For this review, take the finished solid that the model builds, in its own axes (mm). Face numbers are marked on the shaded views. A direction names the side the tool comes from. Give positions to 0.01 mm unless a question says otherwise; leave off trailing zeros. Order: outer loops, then holes, each group sorted by start corner. A loop starts at its lowest first (then second) coordinate and runs counter-clockwise, first axis right, second up.
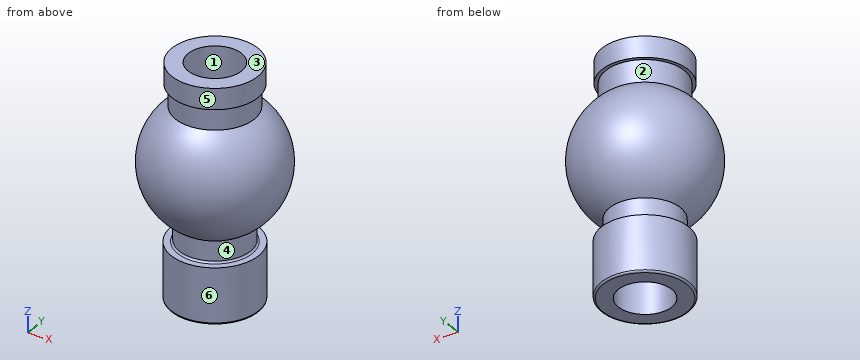
from build123d import *

# Parameters (mm, degrees)
SKETCH1_R           = 2.45
SKETCH1_R_2         = 1.5
BOSS_EXTRUDE1_DEPTH = 3.12
SKETCH2_R           = 1.99
SKETCH2_R_2         = 1.5
BOSS_EXTRUDE2_DEPTH = 1.2
FILLET1_R           = 0.1
CUT_EXTRUDE1_START  = -8.2
SKETCH5_R           = 1.5
CUT_EXTRUDE1_DEPTH  = 8.2
SKETCH6_R           = 2.21
SKETCH6_R_2         = 1.5
BOSS_EXTRUDE3_DEPTH = 1.24
SKETCH7_R           = 2.41
SKETCH7_R_2         = 1.5
BOSS_EXTRUDE4_DEPTH = 1.17


with BuildPart() as part:
    # Sketch1 → Boss-Extrude1 (new body)
    with BuildSketch(Plane.XY):
        with Locations(Location((0, 0, 0), (0, 0, 180))):
            Circle(SKETCH1_R)
        with Locations(Location((0, 0, 0), (0, 0, 180))):
            Circle(SKETCH1_R_2, mode=Mode.SUBTRACT)
    extrude(amount=BOSS_EXTRUDE1_DEPTH)

    # Sketch2 → Boss-Extrude2 (add)
    with BuildSketch(Plane.XY.offset(3.12)):
        Circle(SKETCH2_R)
        with Locations(Location((0, 0, 0), (0, 0, 180))):
            Circle(SKETCH2_R_2, mode=Mode.SUBTRACT)
    extrude(amount=BOSS_EXTRUDE2_DEPTH)

    # Fillet1
    fillet1_edges = [part.edges().sort_by_distance(p)[0] for p in [
        (-1.99, 0, 3.12),
        (2.45, 0, 0),
    ]]
    fillet(fillet1_edges, radius=FILLET1_R)

    # Sketch3 → Revolve1 (revolve)
    with BuildSketch(Plane(origin=(0, 0, 0), x_dir=(0, 0, -1), z_dir=(1, 0, 0))):
        with BuildLine():
            Line((-4.32, 0), (-4.32, 1.99))
            ThreePointArc((-4.32, 1.99), (-7.365617926, 3.747647485), (-10.528014715, 2.21))
            Line((-10.528014715, 2.21), (-10.528014715, 0))
            Line((-10.528014715, 0), (-4.32, 0))
        make_face()
    revolve(axis=Axis((0, 0, 4.32), (0, 0, 1)))

    # Sketch5 → Cut-Extrude1 (cut)
    with BuildSketch(Plane.XY.offset(10.528014715).offset(CUT_EXTRUDE1_START)):
        with Locations(Location((0, 0, 0), (0, 0, 180))):
            Circle(SKETCH5_R)
    extrude(amount=CUT_EXTRUDE1_DEPTH, mode=Mode.SUBTRACT)

    # Sketch6 → Boss-Extrude3 (add)
    with BuildSketch(Plane.XY.offset(10.528014715)):
        with Locations(Location((0, 0, 0), (0, 0, 90))):
            Circle(SKETCH6_R)
        with Locations(Location((0, 0, 0), (0, 0, 180))):
            Circle(SKETCH6_R_2, mode=Mode.SUBTRACT)
    extrude(amount=BOSS_EXTRUDE3_DEPTH)

    # Sketch7 → Boss-Extrude4 (add)
    with BuildSketch(Plane.XY.offset(11.768014715)):
        with Locations(Location((0, 0, 0), (0, 0, 180))):
            Circle(SKETCH7_R)
        with Locations(Location((0, 0, 0), (0, 0, 180))):
            Circle(SKETCH7_R_2, mode=Mode.SUBTRACT)
    extrude(amount=BOSS_EXTRUDE4_DEPTH)


solid = part.part
1) We need section A-A on y = 0. Give the boundary of the cut face in (x, z), then the cut area to 3 significant figures.
Answer sheet:
outline: (-2.45, 0.1) arc R0.1 ccw to (-2.35, 0) - (-1.5, 0) - (-1.5, 12.94) - (-2.41, 12.94) - (-2.41, 11.77) - (-2.21, 11.77) - (-2.21, 10.53) arc R3.75 ccw to (-1.99, 4.32) - (-1.99, 3.22) arc R0.1 cw to (-2.09, 3.12) - (-2.45, 3.12) - close; (1.5, 0) - (2.35, 0) arc R0.1 ccw to (2.45, 0.1) - (2.45, 3.12) - (2.09, 3.12) arc R0.1 cw to (1.99, 3.22) - (1.99, 4.32) arc R3.75 ccw to (2.21, 10.53) - (2.21, 11.77) - (2.41, 11.77) - (2.41, 12.94) - (1.5, 12.94) - close
area: 32.8 mm2
2) We need section D-D on z = 1.25. Give the boundary of the cut face in (x, y), then the cut area to 3 significant figures.
Answer sheet:
outline: circle Ø4.9 at (0, 0); hole circle Ø3 at (0, 0)
area: 11.8 mm2
3) To check wall thickness, follow line 1 (Z direction, x = -2, y = -0.75); line 2 (Y direction, x = -0.75, z = 1.75); line 3 (Y direction, x = 0, z = 5). State the ranges of each line that lie inside material, in increasing order.
Answer sheet:
line 1: z = 0 to 3.12, 4.42 to 12.94
line 2: y = -2.33 to -1.3, 1.3 to 2.33
line 3: y = -2.8 to -1.5, 1.5 to 2.8
4) Tool access review of the marked faces 4, 5 and 6: name each direction out of +Z, -Z, +X, -X, +Y, -Y from which nothing blocks a thin tool from reaching the whole face with its end or side.
Answer sheet:
face 4: none
face 5: +Z
face 6: -Z
5) We need section C-C on z = 12.25. Give the boundary of the cut face in (x, y).
Answer sheet:
outline: circle Ø4.82 at (0, 0); hole circle Ø3 at (0, 0)
6) Clearance check with flat-ended pins moving along their axes: pin 1 (4 mm diameter, centred on x = 0.5, y = 0.5, fed in from +Z); pin 2 (2 mm diameter, centred on x = 0, z = 3.5, fed in from -Y); pin 3 (2 mm diameter, centred on y = 2, z = 2.5, fed in from +X). State where each tip first meets the part, or that it passes through.
Answer sheet:
pin 1: stops at z = 12.94
pin 2: stops at y = -2.45
pin 3: stops at x = 2.24
7) Draft analysis for pull direction X (two halves, no side actions). For the marked faces 1, 2 and 3, state which applies: +X half, -X half, draft (parallel to the pull), parting line (faces both ways), or undercut.
Answer sheet:
face 1: undercut
face 2: parting line
face 3: draft
